CAD build for the part. Positions are in the model's coordinates, mm. Coordinates: 2 decimals unless noted, no trailing zeros. Order: outer loops, then holes, each group sorted by start corner. A loop starts at its lowest first (then second) coordinate and runs counter-clockwise, first axis right, second up. Notation, with made-up numbers: (49.5, 72) - (92.5, 72) arc R18 cw to (92.5, 98) - close; hole circle Ø9 at (-39.5, 79.25). An arc over 180 degrees is marked (long way). Write each question's results on one line, items separated by ' | '. Start each with the question number.
Q1. Pin check, flat tips, straight feed: P1, Ø1.8, axis at x = -51.02, y = 27.22, coming from the +Z side; P2, Ø2.5, axis at x = -51.02, y = -28.76, coming from the -Z side. Stop position of each tip, or through.
Q2. Band-saw the part on A-A, the plane z = 0.35. Count the separate pieces of the cut face and the enclosed holes in it, then the cut area to 3 significant figures.
Q3. Band-saw the part on B-B, the plane y = -10. Write the cut outline in (x, z), then the cut area to 3 significant figures.
Q4. Wall check: probe 1 along Y at (x, z) = (-50.5, 0.7); probe 2 along Y at (x, z) = (-112.5, 1.3); probe 3 along X at (y, z) = (-32, 0.3). Give the ranges that are in metal, low to high.
Q5. Band-saw the part on C-C, the plane x = -91.5. Write the cut outline in (y, z), then the cut area to 3 significant figures.
```python
from build123d import *

# Parameters (mm, degrees)
BOSS_EXTRUDE1_DEPTH = 1.5
SKETCH6_R           = 1
CUT_EXTRUDE1_DEPTH  = 10
FILLET4_R           = 1.5
FILLET5_R           = 3


# Read off the part's stored shape, not the designer's step: AdvancedHole1
with BuildPart() as part:
    # Sketch1 → Boss-Extrude1 (new body)
    with BuildSketch(Plane.XY):
        Polygon((-133.021138037, 63.390093572), (12.778856844, 63.390093572), (12.778856844, -23.568490874), (18.017758559, -33.522553443), (47.405744057, -50.489714781), (27.001354783, -85.831153701), (5.566925134, -73.455979973), (-20.396575573, -64.006038538), (-17.68284447, -56.550123611), (-33.223388364, -53.809906428), (-133.021138037, -53.809906428), align=None)
    extrude(amount=BOSS_EXTRUDE1_DEPTH)

    # Sketch6 → Cut-Extrude1 (cut)
    with BuildSketch(Plane(origin=(0, 0, 0), x_dir=(-1, 0, 0), z_dir=(0, 0, -1))):
        with Locations((126.521138037, 51.256145572)):
            Circle(SKETCH6_R)
        with Locations((108.221138037, -18.975958428)):
            Circle(SKETCH6_R)
        with Locations((51.021138037, -28.759906428)):
            Circle(SKETCH6_R)
        with Locations((51.021138037, 27.224041572)):
            Circle(SKETCH6_R)
        with Locations((1.021138037, 57.990093572)):
            Circle(SKETCH6_R)
        with Locations((1.021138037, -32.009906428)):
            Circle(SKETCH6_R)
        with Locations((12.005086037, -60.259906428)):
            Circle(SKETCH6_R)
        with Locations((-35.744913963, -52.259906428)):
            Circle(SKETCH6_R)
        with Locations((-22.978861963, -73.259906428)):
            Circle(SKETCH6_R)
    extrude(amount=-CUT_EXTRUDE1_DEPTH, mode=Mode.SUBTRACT)

    # AdvancedHole1 outline → AdvancedHole1 (revolve, cut)
    with BuildSketch(Plane(origin=(35.744913963, -52.259906428, 0), x_dir=(1, 0, 0), z_dir=(0, -1, 0))):
        Polygon((2.2, 0), (1, 1.2), (1, 0), align=None)
    revolve(axis=Axis((35.744913963, -52.259906428, 0), (0, 0, 1)), mode=Mode.SUBTRACT)

    # AdvancedHole1 2 outline → AdvancedHole1 2 (revolve, cut)
    with BuildSketch(Plane(origin=(22.978861963, -73.259906428, 0), x_dir=(1, 0, 0), z_dir=(0, -1, 0))):
        Polygon((2.2, 0), (1, 1.2), (1, 0), align=None)
    revolve(axis=Axis((22.978861963, -73.259906428, 0), (0, 0, 1)), mode=Mode.SUBTRACT)

    # AdvancedHole1 3 outline → AdvancedHole1 3 (revolve, cut)
    with BuildSketch(Plane(origin=(-12.005086037, -60.259906428, 0), x_dir=(1, 0, 0), z_dir=(0, -1, 0))):
        Polygon((2.2, 0), (1, 1.2), (1, 0), align=None)
    revolve(axis=Axis((-12.005086037, -60.259906428, 0), (0, 0, 1)), mode=Mode.SUBTRACT)

    # AdvancedHole1 4 outline → AdvancedHole1 4 (revolve, cut)
    with BuildSketch(Plane(origin=(-1.021138037, -32.009906428, 0), x_dir=(1, 0, 0), z_dir=(0, -1, 0))):
        Polygon((2.2, 0), (1, 1.2), (1, 0), align=None)
    revolve(axis=Axis((-1.021138037, -32.009906428, 0), (0, 0, 1)), mode=Mode.SUBTRACT)

    # AdvancedHole1 5 outline → AdvancedHole1 5 (revolve, cut)
    with BuildSketch(Plane(origin=(-51.021138037, -28.759906428, 0), x_dir=(1, 0, 0), z_dir=(0, -1, 0))):
        Polygon((2.2, 0), (1, 1.2), (1, 0), align=None)
    revolve(axis=Axis((-51.021138037, -28.759906428, 0), (0, 0, 1)), mode=Mode.SUBTRACT)

    # AdvancedHole1 6 outline → AdvancedHole1 6 (revolve, cut)
    with BuildSketch(Plane(origin=(-108.221138037, -18.975958428, 0), x_dir=(1, 0, 0), z_dir=(0, -1, 0))):
        Polygon((2.2, 0), (1, 1.2), (1, 0), align=None)
    revolve(axis=Axis((-108.221138037, -18.975958428, 0), (0, 0, 1)), mode=Mode.SUBTRACT)

    # AdvancedHole1 7 outline → AdvancedHole1 7 (revolve, cut)
    with BuildSketch(Plane(origin=(-126.521138037, 51.256145572, 0), x_dir=(1, 0, 0), z_dir=(0, -1, 0))):
        Polygon((2.2, 0), (1, 1.2), (1, 0), align=None)
    revolve(axis=Axis((-126.521138037, 51.256145572, 0), (0, 0, 1)), mode=Mode.SUBTRACT)

    # AdvancedHole1 8 outline → AdvancedHole1 8 (revolve, cut)
    with BuildSketch(Plane(origin=(-51.021138037, 27.224041572, 0), x_dir=(1, 0, 0), z_dir=(0, -1, 0))):
        Polygon((2.2, 0), (1, 1.2), (1, 0), align=None)
    revolve(axis=Axis((-51.021138037, 27.224041572, 0), (0, 0, 1)), mode=Mode.SUBTRACT)

    # AdvancedHole1 9 outline → AdvancedHole1 9 (revolve, cut)
    with BuildSketch(Plane(origin=(-1.021138037, 57.990093572, 0), x_dir=(1, 0, 0), z_dir=(0, -1, 0))):
        Polygon((2.2, 0), (1, 1.2), (1, 0), align=None)
    revolve(axis=Axis((-1.021138037, 57.990093572, 0), (0, 0, 1)), mode=Mode.SUBTRACT)

    # Fillet4
    fillet4_edges = [part.edges().sort_by_distance(p)[0] for p in [
        (-133.021138037, 63.390093572, 0.75),
        (12.778856844, 63.390093572, 0.75),
        (47.405744057, -50.489714781, 0.75),
        (27.001354783, -85.831153701, 0.75),
        (-133.021138037, -53.809906428, 0.75),
    ]]
    fillet(fillet4_edges, radius=FILLET4_R)

    # Fillet5
    fillet5_edges = [part.edges().sort_by_distance(p)[0] for p in [
        (12.778856844, -23.568490874, 0.75),
        (18.017758559, -33.522553443, 0.75),
        (-20.396575573, -64.006038538, 0.75),
        (-17.68284447, -56.550123611, 0.75),
        (-33.223388364, -53.809906428, 0.75),
    ]]
    fillet(fillet5_edges, radius=FILLET5_R)


solid = part.part
```
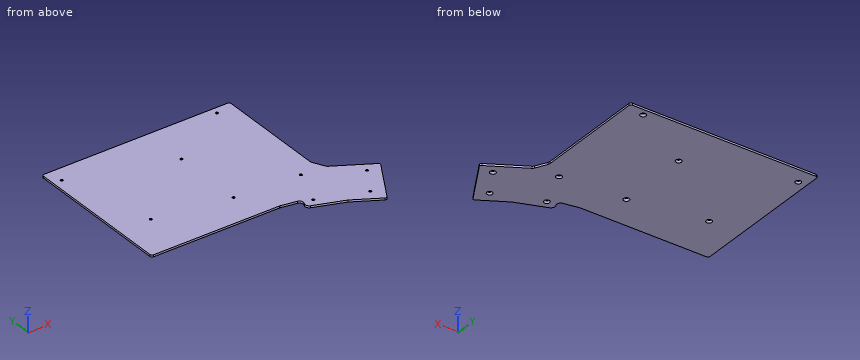
Results below:
1) P1: passes through | P2: stops at z = 0.95
2) separate pieces: 1 | enclosed holes: 9 | area: 18,700 mm²
3) outline: (-133.02, 0) - (12.78, 0) - (12.78, 1.5) - (-133.02, 1.5) - close | area: 219 mm²
4) probe 1: y = -53.81 to -30.17, -27.35 to 25.82, 28.63 to 63.39 | probe 2: y = -53.81 to 63.39 | probe 3: x = -133.02 to -2.92, 0.88 to 17.22
5) outline: (-53.81, 0) - (63.39, 0) - (63.39, 1.5) - (-53.81, 1.5) - close | area: 176 mm²
